Part model, mm, in its own coordinate system. A direction names the side the tool comes from. Round coordinates to 2 decimals unless told otherwise and drop trailing zeros. Loops run counter-clockwise (first coordinate to the right, second up) from the corner with the lowest first, then second, coordinate; pieces in that order, holes last. Notation, with made-up numbers: (22, 50) -> (63, 50) arc R10 ccw to (63, 63) -> close; hole circle Ø7 at (54, -4). An arc over 180 degrees is marked (long way). Use a Markdown table: item, result. Add a question column.
Item 1: Flat gauge pins, fed straight in: pin 1 (2 mm diameter, centred on y = 3.5, z = 32.5, fed in from -X); pin 2 (3 mm diameter, centred on x = 59.9, z = 7.36, fed in from -Y); pin 3 (2 mm diameter, centred on x = 20.5, y = 6, fed in from -Z). Where does each tip first touch, or does it go through?
Item 2: Cut at D-D, the plane x = 16. List the corners of the cut face in (y, z), plus the area to 3 significant figures.
Item 3: Cut at B-B, the plane x = 2.89. List the corners of the cut face in (y, z).
Item 4: Cut at A-A, the plane z = 16.6. List the corners of the cut face in (x, y), plus the area to 3 significant figures.
Item 5: Two-plate mould, pull along X, no slides. Class faces 1 (the face through (2, 5, 32)), 2 (the face through (83.5, 1, 20)), 3 (the face through (33.344, 0.811, 16.383)), 4 (the face through (13, 5, 32)): pulls with the +X half, pulls with the -X half, needs draft (parallel to the pull), parting line crosses it, or undercut.
Item 6: Which spindle directions (+Z, -Z, +X, -X, +Y, -Y) get a long thin tool onto all of the face, cutting with end or side? Do faces 5 (the face through (0, 1, 20)), 6 (the face through (86, 1.6, 22)), 7 (the face through (28, 5, 32)), 8 (the face through (74, 3, 12.2)), 9 (the face through (86, 2.6, 22)). Say none if no direction does.
Item 7: Probe line 1 (X direction, y = 0.3, z = 7.36); line 2 (X direction, y = 6.25, z = 35); line 3 (Y direction, x = 29.5, z = 23.5). List the from-to ranges inside material, lowest first. Write a range as [from, to].
Item 8: Cut at C-C, the plane z = 21. List the corners of the cut face in (x, y), plus the area to 3 significant figures.
```python
from build123d import *

# Parameters (mm, degrees)
SKETCH2_W           = 83.5
SKETCH2_H           = 39
BOSS_EXTRUDE1_DEPTH = 1.6
SKETCH3_W           = 25.5
SKETCH3_H           = 19
BOSS_EXTRUDE2_DEPTH = 1
SKETCH4_W           = 18.466737103
SKETCH4_H           = 19
BOSS_EXTRUDE3_DEPTH = 2.2
SKETCH5_R           = 1
CUT_EXTRUDE1_DEPTH  = 2.2
SKETCH6_W           = 11
SKETCH6_H           = 11
BOSS_EXTRUDE4_DEPTH = 7
SKETCH7_W           = 31
SKETCH7_H           = 15
BOSS_EXTRUDE5_DEPTH = 7.5


with BuildPart() as part:
    # Sketch2 → Boss-Extrude1 (new body)
    with BuildSketch(Plane(origin=(0, 0, 0), x_dir=(1, 0, 0), z_dir=(0, 1, 0))):
        with Locations((41.75, -19.5)):
            Rectangle(SKETCH2_W, SKETCH2_H)
    extrude(amount=BOSS_EXTRUDE1_DEPTH)

    # Sketch3 → Boss-Extrude2 (add)
    with BuildSketch(Plane(origin=(0, 1.6, 0), x_dir=(1, 0, 0), z_dir=(0, 1, 0))):
        with Locations((76.75, -21.7)):
            Rectangle(SKETCH3_W, SKETCH3_H)
    extrude(amount=BOSS_EXTRUDE2_DEPTH)

    # Sketch4 → Boss-Extrude3 (add)
    with BuildSketch(Plane(origin=(0, 2.6, 0), x_dir=(1, 0, 0), z_dir=(0, 1, 0))):
        with Locations((73.233368552, -21.7)):
            Rectangle(SKETCH4_W, SKETCH4_H)
    extrude(amount=BOSS_EXTRUDE3_DEPTH)

    # Sketch5 → Cut-Extrude1 (cut)
    with BuildSketch(Plane(origin=(0, 1.6, 0), x_dir=(1, 0, 0), z_dir=(0, 1, 0))):
        with Locations(Location((59.9, -7.36, 0), (0, 0, 270))):
            Circle(SKETCH5_R)
        with Locations(Location((34.32, -16.6, 0), (0, 0, 270))):
            Circle(SKETCH5_R)
        with Locations(Location((2.89, -12.6, 0), (0, 0, 270))):
            Circle(SKETCH5_R)
    extrude(amount=-CUT_EXTRUDE1_DEPTH, mode=Mode.SUBTRACT)

    # Sketch6 → Boss-Extrude4 (add)
    with BuildSketch(Plane(origin=(0, 1.6, 0), x_dir=(1, 0, 0), z_dir=(0, 1, 0))):
        with Locations((7.5, -31.5)):
            Rectangle(SKETCH6_W, SKETCH6_H)
        with Locations((22.5, -31.5)):
            Rectangle(SKETCH6_W, SKETCH6_H)
    extrude(amount=BOSS_EXTRUDE4_DEPTH)

    # Sketch7 → Boss-Extrude5 (add)
    with BuildSketch(Plane(origin=(0, 0, 0), x_dir=(-1, 0, 0), z_dir=(0, -1, 0))):
        with Locations((-15.3, -29.5)):
            Rectangle(SKETCH7_W, SKETCH7_H)
    extrude(amount=BOSS_EXTRUDE5_DEPTH)


solid = part.part
```
A:
| question | item | result |
|---|---|---|
| 1 | pin 1 | stops at x = 2 |
| 1 | pin 2 | stops at y = 0 |
| 1 | pin 3 | stops at z = 26 |
| 2 | outline | (-7.5, 22) -> (0, 22) -> (0, 0) -> (1.6, 0) -> (1.6, 39) -> (0, 39) -> (0, 37) -> (-7.5, 37) -> close |
| 2 | area | 175 mm^2 |
| 3 | outline | (-7.5, 22) -> (0, 22) -> (0, 13.6) -> (1.6, 13.6) -> (1.6, 26) -> (8.6, 26) -> (8.6, 37) -> (1.6, 37) -> (1.6, 39) -> (0, 39) -> (0, 37) -> (-7.5, 37) -> close; (0, 0) -> (1.6, 0) -> (1.6, 11.6) -> (0, 11.6) -> close |
| 4 | outline | (0, 0) -> (33.32, 0) -> (33.32, 1.6) -> (0, 1.6) -> close; (35.32, 0) -> (83.5, 0) -> (83.5, 1.6) -> (89.5, 1.6) -> (89.5, 2.6) -> (82.47, 2.6) -> (82.47, 4.8) -> (64, 4.8) -> (64, 1.6) -> (35.32, 1.6) -> close |
| 4 | area | 197 mm^2 |
| 5 | face 1 | pulls with the -X half |
| 5 | face 2 | pulls with the +X half |
| 5 | face 3 | undercut |
| 5 | face 4 | undercut |
| 6 | face 5 | +Z, -Z, -X, +Y |
| 6 | face 6 | +Z, -Z, +X, -Y |
| 6 | face 7 | +Z, -Z, +Y |
| 6 | face 8 | -Z, +X, -X, +Y |
| 6 | face 9 | +Z, -Z, +X, +Y |
| 7 | line 1 | x = [0, 58.9], [60.9, 83.5] |
| 7 | line 2 | x = [2, 13], [17, 28] |
| 7 | line 3 | y = [-7.5, 1.6] |
| 8 | outline | (0, 0) -> (83.5, 0) -> (83.5, 1.6) -> (89.5, 1.6) -> (89.5, 2.6) -> (82.47, 2.6) -> (82.47, 4.8) -> (64, 4.8) -> (64, 1.6) -> (0, 1.6) -> close |
| 8 | area | 200 mm^2 |
